The listing builds one solid part. Answer for the finished solid, in the listing's coordinates (mm). Coordinates: 2 decimals unless noted, no trailing zeros. Order: outer loops, then holes, each group sorted by start corner. A loop starts at its lowest first (then second) coordinate and runs counter-clockwise, first axis right, second up. Notation, with made-up numbers: (54.5, 59) - (104.5, 59) arc R11 cw to (104.5, 72) - close; hole circle Ø3 at (12, 76). An arc over 180 degrees is marked (long way). Use one line per item in the form item = value. Start each with the question number.
Item 1: Section A-A, the plane y = 0 is taken. Write down the section's boundary in (x, z), and give its area (4 significant figures).
Item 2: Section C-C, the plane z = 8 is taken. Write down the section's boundary in (x, y), and give its area (3 significant figures).
Item 3: Consider line 1 along Y through (x, z) = (1.05, 0); line 2 along Z through (x, y) = (0.25, -7); line 3 along Z through (x, y) = (1.2, -17.75). Determine where each line is inside the solid, lowest interval first. Write a range as [from, to].
Item 4: Each of these flat-tipped pins is pushed along its axis until it touches: pin 1 Ø2.5 at (y, z) = (17.75, 0) entering from +X; pin 2 Ø1.2 at (y, z) = (0, -17.75) entering from -X. Where does it stop, or does it pass through?
Autodesk Inventor part; units mm, degrees
ref_plane "YZ Plane" through (0, 0, 0) normal (1, 0, 0) x (0, 1, 0)
ref_plane "XZ Plane" through (0, 0, 0) normal (0, 1, 0) x (-1, 0, 0)
ref_plane "XY Plane" through (0, 0, 0) normal (0, 0, 1) x (1, 0, 0)
sketch "Sketch1" plane through (0, 0, 0) normal (1, 0, 0) x (0, 1, 0)
  circle A0 centre (0, 0) radius 16
  circle A1 centre (0, 0) radius 19.5
  dimension "d0" = 32
  dimension "d1" = 39
extrude "Extrusion1" add sketch "Sketch1" along normal blind 2 and the other way blind 2 contours A0
sketch "Sketch2" plane through (2, 0, 0) normal (1, 0, 0) x (0, 0, -1)
  circle A0 centre (0, 0) radius 19.5
  circle A1 centre (0, 0) radius 16
  dimension "d6" = 39
extrude "Extrusion2" add sketch "Sketch2" against normal blind 2
sketch "Sketch3" plane through (-2, 0, 0) normal (-1, 0, 0) x (0, 0, 1)
  circle A0 centre (0, 0) radius 16
  circle A1 centre (0, 0) radius 15
  dimension "d9" = 30
extrude "Extrusion3" cut sketch "Sketch3" against normal blind 10 contours A1
sketch "Sketch5" plane through (0, 0, 0) normal (-1, 0, 0) x (0, 0, 1)
  circle A0 centre (0, 0) radius 17.75
  circle A1 centre (0, 17.75) radius 1
  circle A2 centre (-17.75, 0) radius 1
  circle A3 centre (0, -17.75) radius 1
  circle A4 centre (17.75, 0) radius 1
  dimension "d12" = 35.5
  dimension "d13" = 2
  dimension "d16" = 360
hole "Hole1" at (0, 17.75, 0) at (0, 0, 17.75) at (0, -17.75, 0) at (0, 0, -17.75) direction (1, 0, 0) diameter 2 end through all
sketch "Sketch7" plane through (-2, 0, 0) normal (-1, 0, 0) x (0, 0, 1)
  circle A0 centre (0, 0) radius 15
  circle A1 centre (0, 0) radius 16
extrude "Extrusion4" cut sketch "Sketch7" against normal blind 2
properties part number "base_bearing_holder" material "PET Plastic"
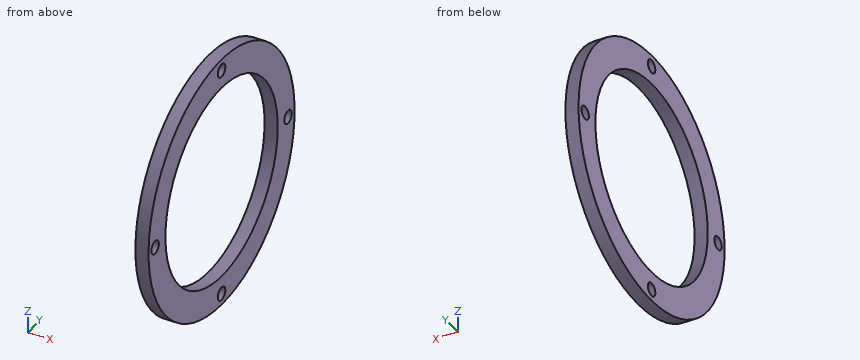
Response:
q1.outline = (0, -19.5) - (2, -19.5) - (2, -18.75) - (0, -18.75) - close; (0, -16.75) - (2, -16.75) - (2, -15) - (0, -15) - close; (0, 15) - (2, 15) - (2, 16.75) - (0, 16.75) - close; (0, 18.75) - (2, 18.75) - (2, 19.5) - (0, 19.5) - close
q1.area = 10.00 mm2
q2.outline = (0, -17.78) - (2, -17.78) - (2, -12.69) - (0, -12.69) - close; (0, 12.69) - (2, 12.69) - (2, 17.78) - (0, 17.78) - close
q2.area = 20.4 mm2
q3.line_1 = [-19.5, -18.75], [-16.75, -15], [15, 16.75], [18.75, 19.5]
q3.line_2 = [-18.2, -13.27], [13.27, 18.2]
q3.line_3 = [-8.07, -1], [1, 8.07]
q4.pin_1 = 2
q4.pin_2 = through
